Check sheet for the modelled part. Datum: model origin and axes. Units: mm. Face numbers are marked on the shaded views. Round coordinates to 2 decimals unless told otherwise and drop trailing zeros. Write each loop counter-clockwise with the first axis right and the second up, starting at its lowest first coordinate (ties: lowest second). Pieces come first, ordered by that corner, then holes.
Item 1: Section check C-C, the plane y = -15.5. Record the cut outline in (x, z), plus the area to 3 significant figures.
Item 2: Section check D-D, the plane y = -21.5. Record the cut outline in (x, z).
Item 3: Material ranges on line 1 along Y through (x, z) = (61.5, -10.25); line 2 along X through (y, z) = (-14.5, -7); line 3 along X through (y, z) = (-5.75, -15.75), recorded low to high.
Item 4: Release check for a two-part mould opening along Z. For the marked faces 1, 2 and 3 record: pulls with the +Z half, pulls with the -Z half, needs draft (parallel to the pull), parting line crosses it, or undercut.
Item 5: Section check B-B, the plane z = -7.5. Record the cut outline in (x, y), plus the area to 3 significant figures.
Item 6: Section check A-A, the plane x = 12.5. Record the cut outline in (y, z), plus the area to 3 significant figures.
from build123d import *

# Parameters (mm, degrees)
F1_DEPTH     = 25
F2_T         = -2.5
F3_R         = 2
F4_T1_DEPTH  = 25
F4_T4_ANGLE  = 90
F4_T6_ANGLE  = 90
F4_T8_ANGLE  = 90
F4_T10_ANGLE = 90


# Not quite as in the source:
# - a fillet or chamfer that OpenCascade refuses, or shapes differently, is made with other operations: its cross-section is extruded or revolved along the edge and cut away or added
# - a shell that OpenCascade refuses in one call is made with other operations: the cavity is built on its own and cut out


with BuildPart() as f1:
    # F0 (on Front) → F1 (new body)
    with BuildSketch(Plane.XZ):
        Polygon((67.4263688624, 0), (-39.5736311376, 0), (-39.5736311376, 5), (-44.5736311376, 5), (-44.5736311376, -20), (72.4263688624, -20), (72.4263688624, 5), (67.4263688624, 5), align=None)
    extrude(amount=F1_DEPTH)

    # F2: a shell. OpenCascade refuses it in one call, so the cavity is built on its own and cut out:
    # the body offset inwards by the wall thickness, plus a prism from it out through each open face.
    f2_core = offset(f1.part, amount=F2_T, kind=Kind.INTERSECTION, mode=Mode.PRIVATE)
    f2_exits = [f2_core.faces().sort_by_distance(p)[0] for p in [
        (13.926369, -12.5, -2.5),
    ]]
    add(f2_core, mode=Mode.SUBTRACT)
    extrude(f2_exits, amount=-F2_T, mode=Mode.SUBTRACT)

    # F3
    f3_edges = [f1.edges().sort_by_distance(p)[0] for p in [
        (-39.573631, -12.5, 5),
        (-44.573631, -12.5, 5),
        (-42.073631, 0, 5),
        (-42.073631, -25, 5),
        (13.926369, -25, 0),
        (-39.573631, -25, 2.5),
        (-44.573631, -25, -7.5),
        (13.926369, -25, -20),
        (72.426369, -25, -7.5),
        (69.926369, -25, 5),
        (67.426369, -25, 2.5),
        (13.926369, 0, 0),
        (-39.573631, 0, 2.5),
        (-44.573631, 0, -7.5),
        (13.926369, 0, -20),
        (72.426369, 0, -7.5),
        (69.926369, 0, 5),
        (67.426369, 0, 2.5),
        (13.926369, -2.5, -17.5),
        (69.926369, -12.5, -17.5),
        (13.926369, -22.5, -17.5),
        (-42.073631, -12.5, -17.5),
        (-42.073631, -22.5, -8.75),
        (-42.073631, -12.5, 0),
        (-42.073631, -2.5, -8.75),
        (69.926369, -12.5, 0),
        (69.926369, -22.5, -8.75),
        (69.926369, -2.5, -8.75),
        (72.426369, -12.5, 5),
        (67.426369, -12.5, 5),
    ]]
    fillet(f3_edges, radius=F3_R)

    # F4: fillet of radius 5 on 2 edges, made by hand

    # F4_s2 → F4_t1 (cut)
    with BuildSketch(Plane.XZ):
        with BuildLine():
            ThreePointArc((67.4263688624, -20), (70.9619027683, -18.5355339059), (72.4263688624, -15))
            Line((72.4263688624, -15), (72.4263688624, -20))
            Line((72.4263688624, -20), (67.4263688624, -20))
        make_face()
        with BuildLine():
            ThreePointArc((-44.5736311376, -15), (-43.1091650435, -18.5355339059), (-39.5736311376, -20))
            Line((-39.5736311376, -20), (-44.5736311376, -20))
            Line((-44.5736311376, -20), (-44.5736311376, -15))
        make_face()
    extrude(amount=F4_T1_DEPTH, mode=Mode.SUBTRACT)

    # F4_s3 → F4_t4 (revolve, cut)
    with BuildSketch(Plane.YZ.offset(-39.5736311376)):
        with BuildLine():
            ThreePointArc((0, -18), (-0.5857864376, -19.4142135624), (-2, -20))
            Line((-2, -20), (0, -20))
            Line((0, -20), (0, -18))
        make_face()
    revolve(axis=Axis((-39.5736311376, 0, -15), (0, 1, 0)), revolution_arc=F4_T4_ANGLE, mode=Mode.SUBTRACT)

    # F4_s5 → F4_t6 (revolve, cut)
    with BuildSketch(Plane.XY.offset(-15)):
        with BuildLine():
            ThreePointArc((-42.5736311376, -25), (-43.9878447, -24.4142135624), (-44.5736311376, -23))
            Line((-44.5736311376, -23), (-44.5736311376, -25))
            Line((-44.5736311376, -25), (-42.5736311376, -25))
        make_face()
    revolve(axis=Axis((-39.5736311376, -25, -15), (0, -1, 0)), revolution_arc=F4_T6_ANGLE, mode=Mode.SUBTRACT)

    # F4_s7 → F4_t8 (revolve, cut)
    with BuildSketch(Plane.XY.offset(-15)):
        with BuildLine():
            ThreePointArc((70.4263688624, 0), (71.8405824248, -0.5857864376), (72.4263688624, -2))
            Line((72.4263688624, -2), (72.4263688624, 0))
            Line((72.4263688624, 0), (70.4263688624, 0))
        make_face()
    revolve(axis=Axis((67.4263688624, 0, -15), (0, 1, 0)), revolution_arc=F4_T8_ANGLE, mode=Mode.SUBTRACT)

    # F4_s9 → F4_t10 (revolve, cut)
    with BuildSketch(Plane.YZ.offset(67.4263688624)):
        with BuildLine():
            ThreePointArc((-25, -18), (-24.4142135624, -19.4142135624), (-23, -20))
            Line((-23, -20), (-25, -20))
            Line((-25, -20), (-25, -18))
        make_face()
    revolve(axis=Axis((67.4263688624, -25, -15), (0, -1, 0)), revolution_arc=F4_T10_ANGLE, mode=Mode.SUBTRACT)


solid = f1.part
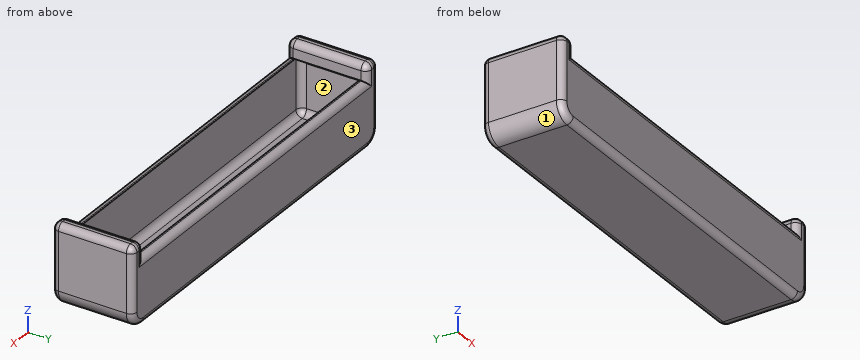
Values found:
1. outline: (-44.57, -15) arc R5 ccw to (-39.57, -20) - (67.43, -20) arc R5 ccw to (72.43, -15) - (72.43, 3) arc R2 ccw to (70.43, 5) - (69.43, 5) arc R2 ccw to (67.43, 3) - (67.43, 0) - (67.93, 0) arc R2 cw to (69.93, -2) - (69.93, -15.5) arc R2 cw to (67.93, -17.5) - (-40.07, -17.5) arc R2 cw to (-42.07, -15.5) - (-42.07, -2) arc R2 cw to (-40.07, 0) - (-39.57, 0) - (-39.57, 3) arc R2 ccw to (-41.57, 5) - (-42.57, 5) arc R2 ccw to (-44.57, 3) - close
1. area: 419 mm2
2. outline: (-44.57, -15) arc R5 ccw to (-39.57, -20) - (67.43, -20) arc R5 ccw to (72.43, -15) - (72.43, 3) arc R2 ccw to (70.43, 5) - (69.43, 5) arc R2 ccw to (67.43, 3) - (67.43, 0) - (67.93, 0) arc R2 cw to (69.66, -1) - (69.66, -15.5) arc R1.73 cw to (67.93, -17.23) - (-40.07, -17.23) arc R1.73 cw to (-41.81, -15.5) - (-41.81, -1) arc R2 cw to (-40.07, 0) - (-39.57, 0) - (-39.57, 3) arc R2 ccw to (-41.57, 5) - (-42.57, 5) arc R2 ccw to (-44.57, 3) - close
3. line 1: y = -25 to -22.5, -2.5 to 0
3. line 2: x = -44.57 to -42.07, 69.93 to 72.43
3. line 3: x = -44.52 to -42.06, 69.91 to 72.37
4. face 1: pulls with the -Z half
4. face 2: undercut
4. face 3: needs draft
5. outline: (-44.57, -23) arc R2 ccw to (-42.57, -25) - (70.43, -25) arc R2 ccw to (72.43, -23) - (72.43, -2) arc R2 ccw to (70.43, 0) - (-42.57, 0) arc R2 ccw to (-44.57, -2) - close; hole (-42.07, -20.5) arc R2 ccw to (-40.07, -22.5) - (67.93, -22.5) arc R2 ccw to (69.93, -20.5) - (69.93, -4.5) arc R2 ccw to (67.93, -2.5) - (-40.07, -2.5) arc R2 ccw to (-42.07, -4.5) - close
5. area: 685 mm2
6. outline: (-25, -18) arc R2 ccw to (-23, -20) - (-2, -20) arc R2 ccw to (0, -18) - (0, -2) arc R2 ccw to (-2, 0) - (-2.5, 0) - (-2.5, -15.5) arc R2 cw to (-4.5, -17.5) - (-20.5, -17.5) arc R2 cw to (-22.5, -15.5) - (-22.5, 0) - (-23, 0) arc R2 ccw to (-25, -2) - close
6. area: 148 mm2
